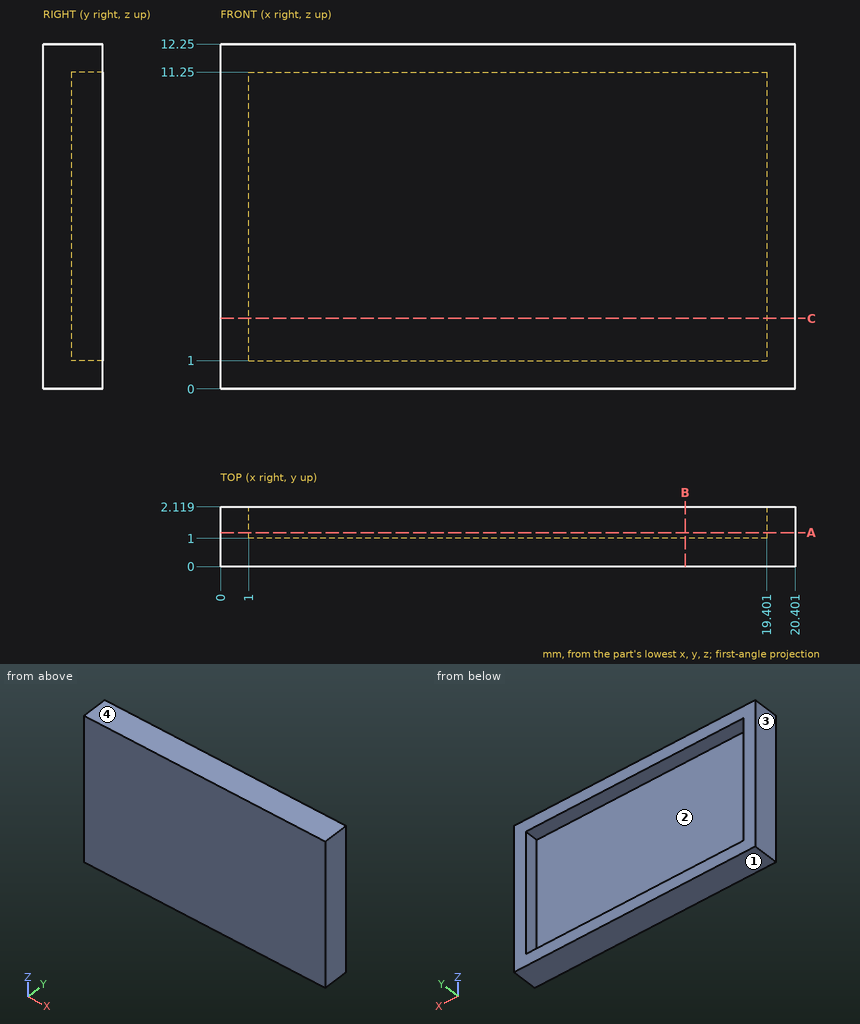
Source: three-view drawing plus pictorial views. Frame: mm from the lowest corner of the part. Round coordinates to 2 decimals unless told otherwise and drop trailing zeros. Loops run counter-clockwise (first coordinate to the right, second up) from the corner with the lowest first, then second, coordinate; pieces in that order, holes last.
1. Section query C-C on z = 2.5. Output: boundary loops of the cut face in (x, y).
2. Section query B-B on x = 16.5. Output: boundary loops of the cut face in (y, z).
3. Mould query, pull axis Z, two halves, no side actions, for the marked faces 1, 2, 3 and 4. Classes: released by +Z, released by -Z, zero draft, split by the parting line, or undercut.
4. Ray query, L1, parallel to X at y = 1.4, z = 10.5; L2, parallel to Z at x = 13, y = 1.1; L3, parallel to Y at x = 7.5, z = 10. Return the intervals inside material, ascending.
5. Section query A-A on y = 1.2. Output: boundary loops of the cut face in (x, z).
6. Contact query for flat-ended pins moving along their axis: pin 1 (1 mm diameter, centred on x = 16.5, z = 7.5, fed in from +Y); pin 2 (0.9 mm diameter, centred on x = 5.5, y = 1.5, fed in from -Z). Output: stop coordinate, or through.
Answers below:
1. outline: (0, 0) - (20.4, 0) - (20.4, 2.12) - (19.4, 2.12) - (19.4, 1) - (1, 1) - (1, 2.12) - (0, 2.12) - close
2. outline: (0, 0) - (2.12, 0) - (2.12, 1) - (1, 1) - (1, 11.25) - (2.12, 11.25) - (2.12, 12.25) - (0, 12.25) - close
3. face 1: released by -Z
3. face 2: undercut
3. face 3: zero draft
3. face 4: released by +Z
4. L1: x = 0 to 1, 19.4 to 20.4
4. L2: z = 0 to 1, 11.25 to 12.25
4. L3: y = 0 to 1
5. outline: (0, 0) - (20.4, 0) - (20.4, 12.25) - (0, 12.25) - close; hole (1, 1) - (19.4, 1) - (19.4, 11.25) - (1, 11.25) - close
6. pin 1: stops at y = 1
6. pin 2: stops at z = 0
